Source: CAD feature listing. Evaluate the final solid. Frame: model axes, mm. A direction names the side the tool comes from. Round coordinates to 2 decimals unless told otherwise and drop trailing zeros. Order: outer loops, then holes, each group sorted by start corner. A loop starts at its lowest first (then second) coordinate and runs counter-clockwise, first axis right, second up. Notation, with made-up numbers: M -31.5,37.5 L -15.5,37.5 A20 ccw -15.5,55.5 Z; hole C 14.5,-37 d5. An arc over 180 degrees is marked long. Answer in a Markdown table with one row per item. Add a question column.
```python
from build123d import *

# Parameters (mm, degrees)
SKETCH114_R   = 1.7
SKETCH114_R_2 = 5
PAD058_DEPTH  = 2
PAD061_DEPTH  = 2
SKETCH119_R   = 4.2
PAD062_DEPTH  = 18
FILLET010_R   = 1


with BuildPart() as part:
    # Sketch114 → Pad058 (new body)
    with BuildSketch(Plane.XY):
        with BuildLine():
            ThreePointArc((-15.5, 21.15), (-19.495153, 19.495153), (-21.15, 15.5))
            Line((-21.15, 15.5), (-21.15, -15.5))
            ThreePointArc((-21.15, -15.5), (-19.495153, -19.495153), (-15.5, -21.15))
            Line((-15.5, -21.15), (15.5, -21.15))
            ThreePointArc((15.5, -21.15), (19.495153, -19.495153), (21.15, -15.5))
            Line((21.15, -15.5), (21.15, 15.500001))
            ThreePointArc((21.15, 15.500001), (19.495153, 19.495154), (15.5, 21.15))
            Line((15.5, 21.15), (-15.5, 21.15))
        make_face()
        with Locations((-15.5, 15.5)):
            Circle(SKETCH114_R, mode=Mode.SUBTRACT)
        with Locations((15.5, 15.5)):
            Circle(SKETCH114_R, mode=Mode.SUBTRACT)
        with Locations((15.5, -15.5)):
            Circle(SKETCH114_R, mode=Mode.SUBTRACT)
        with Locations((-15.5, -15.5)):
            Circle(SKETCH114_R, mode=Mode.SUBTRACT)
        Circle(SKETCH114_R_2, mode=Mode.SUBTRACT)
    extrude(amount=-PAD058_DEPTH)

    # Sketch118 → Pad061 (join)
    with BuildSketch(Plane(origin=(0, 0, -2), x_dir=(1, 0, 0), z_dir=(0, 0, -1))):
        with BuildLine():
            ThreePointArc((7.496486, 25.118361), (0, 28.5), (-7.496486, 25.118361))
            Line((-7.496486, 25.118361), (-11, 21.15))
            Line((11, 21.15), (-11, 21.15))
            Line((7.496486, 25.118361), (11, 21.15))
        make_face()
    extrude(amount=-PAD061_DEPTH)

    # Sketch119 (on Face18 of Pad061) → Pad062 (join)
    with BuildSketch(Plane(origin=(0, 0, -2), x_dir=(1, 0, 0), z_dir=(0, 0, -1))):
        with Locations((0, 18.5)):
            Circle(SKETCH119_R)
    extrude(amount=PAD062_DEPTH)

    # Fillet010
    fillet010_edges = [part.edges().sort_by_distance(p)[0] for p in [
        (-4.2, -18.5, -20),
    ]]
    fillet(fillet010_edges, radius=FILLET010_R)


with BuildPart() as part_1:
    # Body026 placement: moved
    add(part.part.moved(Location((0, 67.5, -103))))


solid = part_1.part
```
(1) Cut plane D-D (z = -107.5). Return loops of the section in (x, y).
(2) Access query for faces 4 (the face through (13, 46.35, -104)), 5 (the face through (0, 49, -123)), 6 (the face through (-0.547, 44.836, -113.381)). Directions: +Z, -Z, +X, -X, +Y, -Y. A direction counts if a zero-diameter tool reaches every point of the face in a straight line with its end or side. Return the directions, or none.
(3) Cut plane C-C (y = 49). Return loops of the section in (x, z), and give its area (3 significant figures).
(4) Line query: line 1 (Y direction, x = 15.5, z = -104.05); line 2 (Y direction, x = 0, z = -104.3); line 3 (X direction, y = 81.5, z = -104.75). Output: solid intervals per line, ascending. Write a range as from..to.
(5) Cut plane A-A (x = 0). Return loops of the section in (y, z).
(6) Pin query (flat end, axial travel): pin 1 (6 mm diameter, centred on x = 0, y = 67.5, fed in from +Z); pin 2 (12 mm diameter, centred on x = -2.5, z = -120, fed in from +Y); pin 3 (0.6 mm diameter, centred on x = -13.5, z = -103.5, fed in from -Y); pin 4 (6 mm diameter, centred on x = 13, z = -106.5, fed in from +Y). Return the tip coordinate at first contact, or that it passes through.
(7) Cut plane B-B (y = 67.5). Return loops of the section in (x, z), and give its area (3 significant figures).
(8) Draft query along X for faces 1 (the face through (-13, 46.35, -104)), 2 (the face through (19.45, 47.96, -103.99)), 3 (the face through (16.3, 81.5, -104)). Return one class per face: +X half, -X half, draft (parallel to the pull), parting line (faces both ways), or undercut.
Answer list:
| question | item | result |
|---|---|---|
| 1 | outline | C 0,49 d8.4 |
| 2 | face 4 | +Z, -Z, +X, -Y |
| 2 | face 5 | -Z, +X, -X, +Y, -Y |
| 2 | face 6 | -Z |
| 3 | outline | M -20.29,-105 L -4.2,-105 L -4.2,-122 A1 ccw -3.2,-123 L 3.2,-123 A1 ccw 4.2,-122 L 4.2,-105 L 20.29,-105 L 20.29,-103 L -20.29,-103 Z |
| 3 | area | 232 mm² |
| 4 | line 1 | 46.35..50.3, 53.7..81.3, 84.7..88.65 |
| 4 | line 2 | 39..62.5, 72.5..88.65 |
| 4 | line 3 | -21.15..-16.3, -14.7..14.7, 16.3..21.15 |
| 5 | outline | M 39,-105 L 44.8,-105 L 44.8,-122 A1 ccw 45.8,-123 L 52.2,-123 A1 ccw 53.2,-122 L 53.2,-105 L 62.5,-105 L 62.5,-103 L 39,-103 Z; M 72.5,-105 L 88.65,-105 L 88.65,-103 L 72.5,-103 Z |
| 6 | pin 1 | through |
| 6 | pin 2 | y = 53.2 |
| 6 | pin 3 | y = 46.35 |
| 6 | pin 4 | y = 88.65 |
| 7 | outline | M -21.15,-105 L -5,-105 L -5,-103 L -21.15,-103 Z; M 5,-105 L 21.15,-105 L 21.15,-103 L 5,-103 Z |
| 7 | area | 64.6 mm² |
| 8 | face 1 | draft |
| 8 | face 2 | +X half |
| 8 | face 3 | undercut |
